Autodesk Inventor part; units mm, degrees
ref_plane "YZ Plane" through (0, 0, 0) normal (1, 0, 0) x (0, 1, 0)
ref_plane "XZ Plane" through (0, 0, 0) normal (0, 1, 0) x (-1, 0, 0)
ref_plane "XY Plane" through (0, 0, 0) normal (0, 0, 1) x (1, 0, 0)
sketch "Sketch1" plane through (0, 0, 0) normal (0, 0, 1) x (1, 0, 0)
  line L0 (0, 0) -> (0, 12.7)
  line L1 (0, 12.7) -> (25.4, 12.7)
  line L2 (25.4, 12.7) -> (25.4, 0)
  line L3 (25.4, 0) -> (0, 0)
  dimension "d0" = 12.7
  dimension "d1" = 25.4
extrude "Extrusion1" add sketch "Sketch1" against normal blind 25.4
sketch "Sketch2" plane through (0, 12.7, 0) normal (0, 1, 0) x (1, 0, 0)
  line L0 (0, 0) -> (12.7, 0) construction
  line L1 (0, 0) -> (25.4, 0) construction
  line L2 (12.7, 0) -> (12.7, 12.7) construction
  circle A0 centre (12.7, 12.7) radius 6.35
  dimension "d4" = 12.7
  dimension "d5" = 12.7
extrude "Extrusion2" cut sketch "Sketch2" against normal blind 15.875
sketch "Sketch3" plane through (0, 12.7, 0) normal (0, 1, 0) x (1, 0, 0)
  point P0 (0, 0)
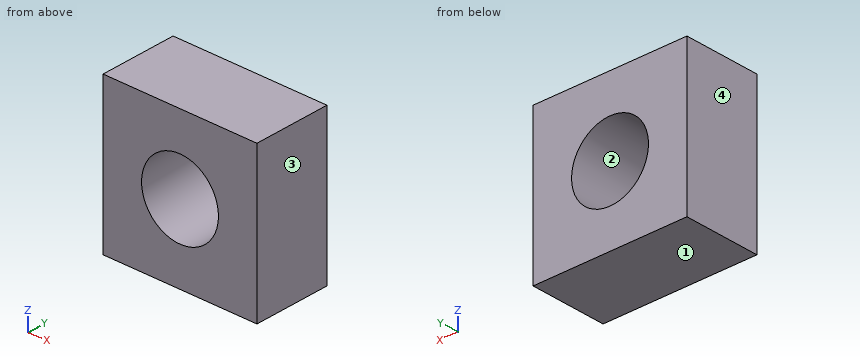
The listing builds one solid part. Answer for the finished solid, in the listing's coordinates (mm). Face numbers are marked on the shaded views. Coordinates: 2 decimals unless noted, no trailing zeros. Write each loop counter-clockwise with the first axis right and the second up, starting at its lowest first coordinate (ties: lowest second). Pieces come first, ordered by that corner, then holes. Notation, with made-up numbers: (42.25, -13.75) - (53.25, -13.75) arc R24 cw to (53.25, -3.75) - close; hole circle Ø3 at (73, 30.25). An arc over 180 degrees is marked (long way). Put each result on its own line as item: value.
1. Determine the mould class of the marked faces 1, 2, 3 and 4 for opening direction X: pulls with the +X half, pulls with the -X half, needs draft (parallel to the pull), parting line crosses it, or undercut.
Answer sheet:
face 1: needs draft
face 2: undercut
face 3: pulls with the +X half
face 4: pulls with the -X half
2. The part is cut by section C-C on y = 1. Give the vertices of the cut face in (x, z).
Answer sheet:
outline: (0, -25.4) - (25.4, -25.4) - (25.4, 0) - (0, 0) - close; hole circle Ø12.7 at (12.7, -12.7)
3. Find the intervals of material crossed by line 1 along X through (y, z) = (7.75, -12.7); line 2 along Z through (x, y) = (12.7, 3); line 3 along Z through (x, y) = (10, 10.75), in increasing order. Write a range as from..to.
Answer sheet:
line 1: x = 0..6.35, 19.05..25.4
line 2: z = -25.4..-19.05, -6.35..0
line 3: z = -25.4..-18.45, -6.95..0
4. The part is cut by section B-B on z = -12.7. Give the vertices of the cut face in (x, y).
Answer sheet:
outline: (0, 0) - (6.35, 0) - (6.35, 12.7) - (0, 12.7) - close; (19.05, 0) - (25.4, 0) - (25.4, 12.7) - (19.05, 12.7) - close
5. The part is cut by section A-A on x = 12.7. Give the vertices of the cut face in (y, z).
Answer sheet:
outline: (0, -25.4) - (12.7, -25.4) - (12.7, -19.05) - (0, -19.05) - close; (0, -6.35) - (12.7, -6.35) - (12.7, 0) - (0, 0) - close
6. A flat-ended cylindrical pin translates along its axis: pin 1 Ø2 at (x, z) = (6, -23) entering from -Y. Find the tip coordinate at first contact, or state that the pin passes through.
Answer sheet:
pin 1: stops at y = 0
